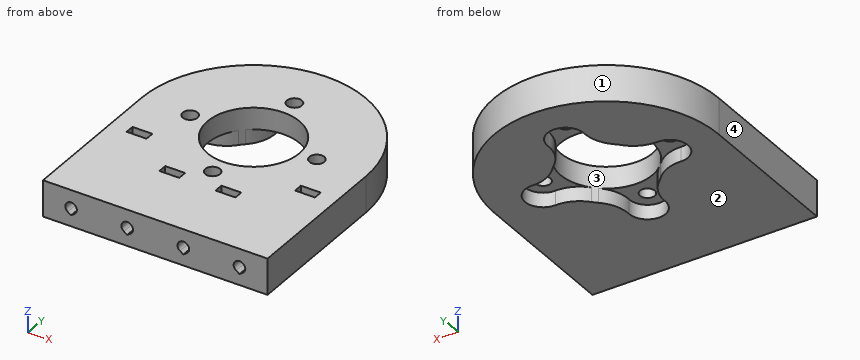
from build123d import *

# Parameters (mm, degrees)
SKETCH1_R                = 12.702118755
BOSS_EXTRUDE1_DEPTH      = 10
SKETCH1_3_R              = 5
CUT_EXTRUDE1_DEPTH       = 4
SKETCH1_4_R              = 2.05
CUT_EXTRUDE3_DEPTH       = 80.937475567
CUT_EXTRUDE3_DEPTH_BACK  = 80.937475567
FILLET1_R                = 10
CUT_EXTRUDE12_START      = -5
SKETCH3_W                = 5.5
SKETCH3_H                = 2.5
CUT_EXTRUDE12_DEPTH      = 80.937475709
CUT_EXTRUDE12_DEPTH_BACK = 2.75
CUT_EXTRUDE13_DEPTH      = 31.5
CUT_EXTRUDE14_DEPTH      = 21.5


with BuildPart() as part:
    # Sketch1 → Boss-Extrude1 (new body)
    with BuildSketch(Plane(origin=(0, 0, 0), x_dir=(0, 1, 0), z_dir=(0, 0, 1))):
        with BuildLine():
            Line((0, 31), (0, -31))
            Line((0, -31), (42, -31))
            ThreePointArc((42, -31), (73, 0), (42, 31))
            Line((42, 31), (0, 31))
        make_face()
        with Locations(Location((42, 0, 0), (0, 0, 270))):
            Circle(SKETCH1_R, mode=Mode.SUBTRACT)
    extrude(amount=BOSS_EXTRUDE1_DEPTH)

    # Sketch1<3> → Cut-Extrude1 (cut)
    with BuildSketch(Plane(origin=(0, 0, 0), x_dir=(0, 1, 0), z_dir=(0, 0, 1))):
        with Locations((59.5, 0)):
            Circle(SKETCH1_3_R)
        with Locations((42, -17.5)):
            Circle(SKETCH1_3_R)
        with Locations((24.5, 0)):
            Circle(SKETCH1_3_R)
        with Locations((42, 17.5)):
            Circle(SKETCH1_3_R)
    extrude(amount=CUT_EXTRUDE1_DEPTH, mode=Mode.SUBTRACT)

    # Sketch1<4> → Cut-Extrude3 (cut, two sides)
    with BuildSketch(Plane(origin=(0, 0, 0), x_dir=(0, 1, 0), z_dir=(0, 0, 1))) as cut_extrude3_sk:
        with Locations(Location((59.5, 0, 0), (0, 0, 270))):
            Circle(SKETCH1_4_R)
        with Locations(Location((42, -17.5, 0), (0, 0, 270))):
            Circle(SKETCH1_4_R)
        with Locations(Location((24.5, 0, 0), (0, 0, 270))):
            Circle(SKETCH1_4_R)
        with Locations(Location((42, 17.5, 0), (0, 0, 270))):
            Circle(SKETCH1_4_R)
    extrude(amount=CUT_EXTRUDE3_DEPTH, mode=Mode.SUBTRACT)
    extrude(cut_extrude3_sk.sketch, amount=-CUT_EXTRUDE3_DEPTH_BACK, mode=Mode.SUBTRACT)

    # Fillet1
    fillet1_edges = [part.edges().sort_by_distance(p)[0] for p in [
        (-1.197579289, 29.354462261, 2),
        (1.197579289, 29.354462261, 2),
        (-12.645537739, 43.197579289, 2),
        (-12.645537739, 40.802420711, 2),
        (1.197579289, 54.645537739, 2),
        (-1.197579289, 54.645537739, 2),
        (12.645537739, 40.802420711, 2),
        (12.645537739, 43.197579289, 2),
    ]]
    fillet(fillet1_edges, radius=FILLET1_R)

    # Sketch3 → Cut-Extrude12 (cut, two sides)
    with BuildSketch(Plane.XY.offset(10).offset(CUT_EXTRUDE12_START)) as cut_extrude12_sk:
        with Locations((-23.25, 29.25)):
            Rectangle(SKETCH3_W, SKETCH3_H)
        with Locations((-7.75, 19.25)):
            Rectangle(SKETCH3_W, SKETCH3_H)
        with Locations((7.75, 19.25)):
            Rectangle(SKETCH3_W, SKETCH3_H)
        with Locations((23.25, 29.25)):
            Rectangle(SKETCH3_W, SKETCH3_H)
    extrude(amount=CUT_EXTRUDE12_DEPTH, mode=Mode.SUBTRACT)
    extrude(cut_extrude12_sk.sketch, amount=-CUT_EXTRUDE12_DEPTH_BACK, mode=Mode.SUBTRACT)

    # Sketch2 → Cut-Extrude13 (cut)
    with BuildSketch(Plane.XZ):
        with BuildLine():
            Line((-22.332277702, 3.689356729), (-23.25, 3.046760658))
            Line((-23.25, 3.046760658), (-24.167722298, 3.689356729))
            ThreePointArc((-24.167722298, 3.689356729), (-23.25, 6.6), (-22.332277702, 3.689356729))
        make_face()
        with BuildLine():
            Line((22.332277702, 3.689356729), (23.25, 3.046760658))
            Line((23.25, 3.046760658), (24.167722298, 3.689356729))
            ThreePointArc((24.167722298, 3.689356729), (23.25, 6.6), (22.332277702, 3.689356729))
        make_face()
    extrude(amount=-CUT_EXTRUDE13_DEPTH, mode=Mode.SUBTRACT)

    # Sketch2<3> → Cut-Extrude14 (cut)
    with BuildSketch(Plane.XZ):
        with BuildLine():
            Line((-8.667722298, 3.689356729), (-7.75, 3.046760658))
            Line((-7.75, 3.046760658), (-6.832277702, 3.689356729))
            ThreePointArc((-6.832277702, 3.689356729), (-7.75, 6.6), (-8.667722298, 3.689356729))
        make_face()
        with BuildLine():
            Line((6.832277702, 3.689356729), (7.75, 3.046760658))
            Line((7.75, 3.046760658), (8.667722298, 3.689356729))
            ThreePointArc((8.667722298, 3.689356729), (7.75, 6.6), (6.832277702, 3.689356729))
        make_face()
    extrude(amount=-CUT_EXTRUDE14_DEPTH, mode=Mode.SUBTRACT)


solid = part.part
Work out the finished part from the listing and answer in its coordinate system (mm). Face numbers are marked on the shaded views. Round coordinates to 2 decimals unless told otherwise and drop trailing zeros. Loops run counter-clockwise (first coordinate to the right, second up) from the corner with the lowest first, then second, coordinate; pieces in that order, holes last. Notation, with made-up numbers: M 17.5,-32 L 41.5,-32 A20 ccw 41.5,2 Z; hole C 56,50.25 d1. An arc over 180 degrees is marked long. One line per question, with ' | ' between items. Start each with the question number.
(1) Find the intervals of material crossed by line 1 (X direction, y = 21.35, z = 5); line 2 (Y direction, x = 0, z = 7.5); line 3 (Z direction, x = 23.25, y = 12.25), in increasing order.
(2) A cutting plane is placed at C-C on y = 68.5. Write down the section's boundary in (x, z), plus the area to 3 significant figures.
(3) A cutting plane is placed at A-A on z = 9. Give the number of separate pieces and of enclosed holes in the cut face, plus the area to 3 significant figures.
(4) For a pull along X with two mould halves and no side action, classify the marked faces 1, 2, 3 and 4 as released by +X, released by -X, zero draft, split by the parting line, or undercut.
(5) Flat-ended cylindrical pins translate along their axes: pin 1 Ø2.5 at (x, z) = (-23.25, 5) entering from -Y; pin 2 Ø1.2 at (x, y) = (-24, 29.5) entering from +Z; pin 3 Ø6.5 at (x, y) = (-17.5, 42) entering from -Z. Find the tip coordinate at first contact, or state that the pin passes through.
(6) A cutting plane is placed at B-B on x = 3.5. Write down the section's boundary in (y, z).
Geometry check:
1) line 1: x = -31 to -24.85, -21.65 to -9.35, -6.15 to 6.15, 9.35 to 21.65, 24.85 to 31 | line 2: y = 0 to 22.45, 26.55 to 29.3, 54.7 to 57.45, 61.55 to 73 | line 3: z = 0 to 3.05, 6.6 to 10
2) outline: M -16.09,0 L 16.09,0 L 16.09,10 L -16.09,10 Z | area: 322 mm²
3) separate pieces: 1 | enclosed holes: 9 | area: 3,500 mm²
4) face 1: split by the parting line | face 2: zero draft | face 3: undercut | face 4: released by -X
5) pin 1: stops at y = 31.5 | pin 2: stops at z = 2.25 | pin 3: stops at z = 4
6) outline: M 0,0 L 20.93,0 L 20.93,4 L 29.79,4 L 29.79,10 L 0,10 Z; M 54.21,4 L 63.07,4 L 63.07,0 L 72.8,0 L 72.8,10 L 54.21,10 Z
